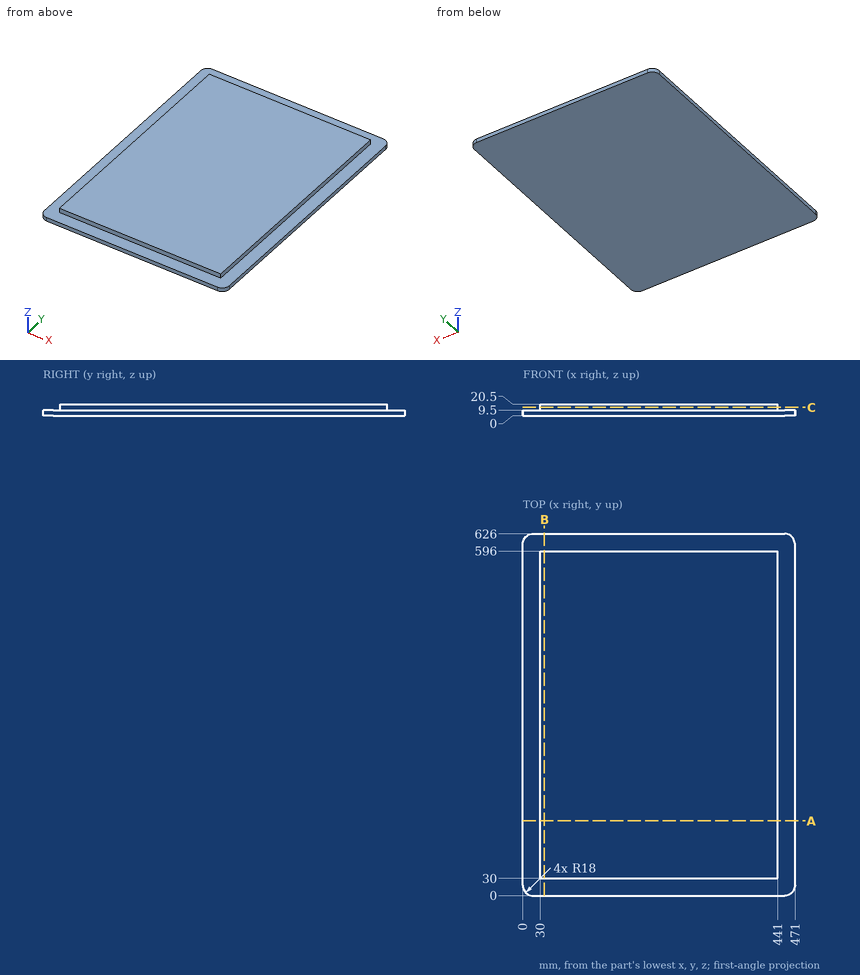
Here's the drawing with two shaded views (mm, measured from the low corner). I have some questions. Give positions to 0.01 mm unless a question says otherwise; leave off trailing zeros. Order: outer loops, then holes, each group sorted by start corner. A loop starts at its lowest first (then second) coordinate and runs counter-clockwise, first axis right, second up. Notation, with made-up numbers: M 84,67.5 L 143,67.5 A23 ccw 143,89.5 Z; hole C 74,21.5 d1. An arc over 180 degrees is marked long. One line per question, with ' | ' between items.
Item 1: Suppose I cut it at A-A, the plane y = 129.5. Write out the boundary of the cut face in (x, z), then the cut area to 3 significant figures.
Answer block:
outline: M 0,0 L 471,0 L 471,9.5 L 441,9.5 L 441,20.5 L 30,20.5 L 30,9.5 L 0,9.5 Z | area: 9,000 mm2
Item 2: I'm going to push flat-ended pins straight in: pin 1 Ø12 at (y, z) = (225.5, 17.5) entering from +X; pin 2 Ø3.5 at (x, z) = (139.5, 15.5) entering from -Y; pin 3 Ø12 at (x, z) = (322.5, 16.5) entering from +Y. Where does each tip first touch, or does it pass through?
Answer block:
pin 1: stops at x = 441 | pin 2: stops at y = 30 | pin 3: stops at y = 596
Item 3: Suppose I cut it at C-C, the plane z = 14.75. Write out the boundary of the cut face in (x, y), then the cut area to 3 significant figures.
Answer block:
outline: M 30,30 L 441,30 L 441,596 L 30,596 Z | area: 233,000 mm2
Item 4: Suppose I cut it at B-B, the plane x = 37.5. Write out the boundary of the cut face in (y, z), then the cut area to 3 significant figures.
Answer block:
outline: M 0,0 L 626,0 L 626,9.5 L 596,9.5 L 596,20.5 L 30,20.5 L 30,9.5 L 0,9.5 Z | area: 12,200 mm2
Item 5: Please list where these lines run through material, in increasing order: L1, parallel to X at y = 429, z = 13.5; L2, parallel to Y at x = 106, z = 18.25.
Answer block:
L1: x = 30 to 441 | L2: y = 30 to 596
